The model under review builds one solid part; all positions refer to its coordinate system, in mm. Coordinates: 2 decimals unless noted, no trailing zeros. Write each loop counter-clockwise with the first axis right and the second up, starting at its lowest first coordinate (ties: lowest second). Pieces come first, ordered by that corner, then holes. Notation, with made-up numbers: (58, 30) -> (105, 30) arc R22 ccw to (105, 50) -> close; hole circle Ø3 at (-22.75, 82.25). An arc over 180 degrees is marked (long way). Put each result on its own line as item: value. Start each with the question number.
from build123d import *

# Parameters (mm, degrees)
F0_R     = 13.49375
F0_R_2   = 11
F1_DEPTH = 6.35
F2_R     = 1.27
F3_R     = 1.27


with BuildPart() as f1:
    # F0 (on Top) → F1 (new body)
    with BuildSketch(Plane.XY):
        Circle(F0_R)
        Circle(F0_R_2, mode=Mode.SUBTRACT)
    extrude(amount=F1_DEPTH)

    # F2
    f2_edges = [f1.edges().sort_by_distance(p)[0] for p in [
        (-13.49375, 0, 0),
    ]]
    fillet(f2_edges, radius=F2_R)

    # F3
    f3_edges = [f1.edges().sort_by_distance(p)[0] for p in [
        (-13.49375, 0, 6.35),
    ]]
    fillet(f3_edges, radius=F3_R)


solid = f1.part
1. Insertion check: P1, Ø3, axis at x = 3.5, z = 4.5, coming from the -Y side; P2, Ø12, axis at x = 0.5, y = -1.5, coming from the +Z side; P3, Ø1.5, axis at y = -9.5, z = 5, coming from the -X side; P4, Ø1, axis at x = -6.5, z = 2.5, coming from the -Y side. Each pin has a flat end and moves straight along its axis. Give the tip position at first contact, or say it passes through.
2. Consider section C-C on z = 0.5. State the section outline as (x, y) points, then the cut area to 3 significant figures.
3. Consider section B-B on z = 2.5. State the section outline as (x, y) points.
4. Wall thickness on line 1 (Y direction, x = 0, z = 4.25); line 2 (Y direction, x = 2, z = 2.5); line 3 (X direction, y = 9.5, z = 2): over which ranges is each line inside the solid? List them lowest first. Write a range as from..to.
5. The part is to be moulded in two halves that separate along X. For faces 1 (the cylindrical face through (-9.945, 9.12, 3.148)), 2 (the flat face through (-10, 5, 0)), 3 (the cylindrical face through (-2.38, -10.74, 3.13)), say which applies: released by +X, released by -X, zero draft, split by the parting line, or undercut.
6. Consider section A-A on y = 0. State the section outline as (x, z) points.
Output values:
1. P1: stops at y = -13.34
1. P2: passes through
1. P3: stops at x = -10.27
1. P4: stops at y = -12.09
2. outline: circle Ø26.47 at (0, 0); hole circle Ø22 at (0, 0)
2. area: 170 mm^2
3. outline: circle Ø26.99 at (0, 0); hole circle Ø22 at (0, 0)
4. line 1: y = -13.49..-11, 11..13.49
4. line 2: y = -13.34..-10.82, 10.82..13.34
4. line 3: x = -9.58..-5.55, 5.55..9.58
5. face 1: split by the parting line
5. face 2: zero draft
5. face 3: undercut
6. outline: (-13.49, 1.27) arc R1.27 ccw to (-12.22, 0) -> (-11, 0) -> (-11, 6.35) -> (-12.22, 6.35) arc R1.27 ccw to (-13.49, 5.08) -> close; (11, 0) -> (12.22, 0) arc R1.27 ccw to (13.49, 1.27) -> (13.49, 5.08) arc R1.27 ccw to (12.22, 6.35) -> (11, 6.35) -> close
